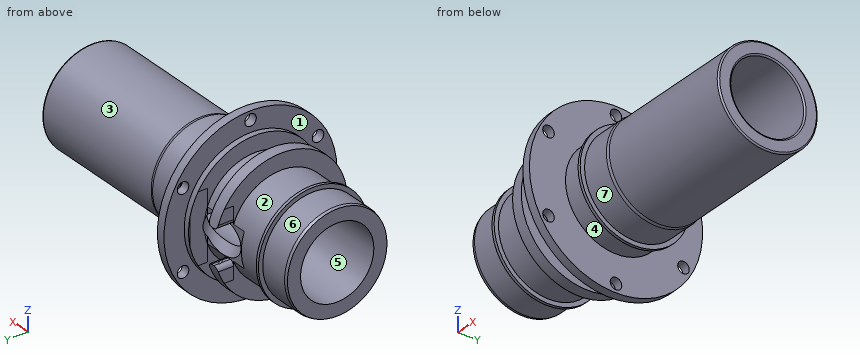
from build123d import *
from build123d.topology import SkipClean

# Parameters (mm, degrees)
SKETCH2_R          = 2
CUT_EXTRUDE1_DEPTH = 92.660037639
CUT_EXTRUDE2_DEPTH = 6.025391911


# Read off the part's stored shape, not the designer's step: Cut-Extrude2
with BuildPart() as part:
    # Sketch1 → Revolve1 (revolve)
    with BuildSketch(Plane.XY, mode=Mode.PRIVATE) as revolve1_sk:
        with BuildLine():
            Line((-1.5, 17.5), (6.5, 17.5))
            Line((6.5, 17.5), (6.5, 23))
            Line((6.5, 23), (8.5, 23))
            Line((8.5, 23), (8.5, 30))
            Line((8.5, 30), (11.5, 30))
            Line((11.5, 30), (11.5, 17.5))
            Line((11.5, 17.5), (19.25, 17.5))
            Line((19.25, 17.5), (19.25, 19))
            Line((19.25, 19), (20.25, 19))
            Line((20.25, 19), (20.25, 17.5))
            Line((20.25, 17.5), (30.25, 17.5))
            Line((30.25, 17.5), (31.25, 17.25))
            Line((31.25, 17.25), (80.75, 17.25))
            ThreePointArc((80.75, 17.25), (81.103553391, 17.103553391), (81.25, 16.75))
            Line((81.25, 16.75), (81.25, 13.2))
            ThreePointArc((81.25, 13.2), (81.103553391, 12.846446609), (80.75, 12.7))
            Line((80.75, 12.7), (-31.25, 12.7))
            Line((-31.25, 12.7), (-31.25, 17.25))
            Line((-31.25, 17.25), (-30.25, 17.5))
            Line((-30.25, 17.5), (-20.25, 17.5))
            Line((-20.25, 17.5), (-20.25, 19))
            Line((-20.25, 19), (-19.25, 19))
            Line((-19.25, 19), (-19.25, 17.5))
            Line((-19.25, 17.5), (-5.5, 17.5))
            Line((-5.5, 17.5), (-5.5, 23))
            Line((-5.5, 23), (-1.5, 23))
            Line((-1.5, 23), (-1.5, 17.5))
        make_face()
    revolve(revolve1_sk.sketch.rotate(Axis((-31.25, 0, 0), (1, 0, 0)), 180), axis=Axis((-31.25, 0, 0), (1, 0, 0)))

    # Sketch2 → Cut-Extrude1 (cut, through all)
    with BuildSketch(Plane(origin=(0, 0, 0), x_dir=(0, 0, -1), z_dir=(1, 0, 0))):
        with Locations(Location((27, 0, 0), (0, 0, 270))):
            Circle(SKETCH2_R)
        with Locations(Location((13.5, -23.382685902, 0), (0, 0, 270))):
            Circle(SKETCH2_R)
        with Locations(Location((-13.5, -23.382685902, 0), (0, 0, 270))):
            Circle(SKETCH2_R)
        with Locations(Location((-27, 0, 0), (0, 0, 270))):
            Circle(SKETCH2_R)
        with Locations(Location((-13.5, 23.382685902, 0), (0, 0, 270))):
            Circle(SKETCH2_R)
        with Locations(Location((13.5, 23.382685902, 0), (0, 0, 270))):
            Circle(SKETCH2_R)
    extrude(amount=CUT_EXTRUDE1_DEPTH, mode=Mode.SUBTRACT)

    # Sketch3 → Cut-Revolve1 (revolve, cut)
    with BuildSketch(Plane.XY):
        Polygon((16, 0), (-16.947446606, 32.947446606), (-21.190087293, 28.704805919), (11.757359313, -4.242640687), align=None)
    revolve(axis=Axis((-23.931199794, 39.931199794, 0), (0.7071067811865516, -0.7071067811865436, 0)), mode=Mode.SUBTRACT)

    # Cut-Extrude2 outline → Cut-Extrude2 (cut)
    with SkipClean():  # the faces are left unmerged after this step: merging them gives an invalid solid
        with BuildSketch(Plane(origin=(0, 16.455853693, 0), x_dir=(1, 0, 0), z_dir=(0, 1, 0))):
            with BuildLine():
                Line((-2.992126028, 5.992167254), (-3.992126028, 5.986917867))
                ThreePointArc((-3.992126028, 5.986917867), (-5.057872639, 6.423456803), (-5.5, 7.4868972))
                Line((-5.5, 7.4868972), (-5.5, 11.85382039))
                Line((-5.5, 11.85382039), (-10.416830721, 11.85382039))
                Line((-10.416830721, 11.85382039), (-10.416830721, 5.95439999))
                Line((-10.416830721, 5.95439999), (-10.416830721, -5.95439999))
                Line((-10.416830721, -5.95439999), (-10.416830721, -11.85382039))
                Line((-10.416830721, -11.85382039), (-5.5, -11.85382039))
                Line((-5.5, -11.85382039), (-5.5, -7.4868972))
                ThreePointArc((-5.5, -7.4868972), (-5.057872639, -6.423456803), (-3.992126028, -5.986917867))
                Line((-3.992126028, -5.986917867), (-2.992126028, -5.992167254))
                ThreePointArc((-2.992126028, -5.992167254), (-1.936559603, -6.434273947), (-1.5, -7.492146587))
                Line((-1.5, -7.492146587), (-1.5, -11.85382039))
                Line((-1.5, -11.85382039), (6.5, -11.85382039))
                Line((6.5, -11.85382039), (6.5, 11.85382039))
                Line((6.5, 11.85382039), (-1.5, 11.85382039))
                Line((-1.5, 11.85382039), (-1.5, 7.492146587))
                ThreePointArc((-1.5, 7.492146587), (-1.936559603, 6.434273947), (-2.992126028, 5.992167254))
            make_face()
        extrude(amount=CUT_EXTRUDE2_DEPTH, mode=Mode.SUBTRACT)


solid = part.part
Part model, mm, in its own coordinate system. Face numbers are marked on the shaded views. A direction names the side the tool comes from. Coordinates: 2 decimals unless noted, no trailing zeros. Order: outer loops, then holes, each group sorted by start corner. A loop starts at its lowest first (then second) coordinate and runs counter-clockwise, first axis right, second up. Notation, with made-up numbers: M 12,-29.75 L 42,-29.75 A13 cw 42,-22.75 Z; hole C 50.5,-12 d3. An arc over 180 degrees is marked long. Use a Markdown table: item, result.
(1) Cut at B-B on x = 41.5. Write the cut outline in (y, z).
A:
| item | result |
|---|---|
| outline | C 0,0 d34.5; hole C 0,0 d25.4 |
(2) Probe L1, parallel to Z at x = 10.35, y = 0; L2, parallel to X at y = 19.5, z = 8.5; L3, parallel to Z at x = 35.5, y = 0. List the from-to ranges inside material, lowest first.
A:
| item | result |
|---|---|
| L1 | z = -30 to -29, -25 to -12.7, 12.7 to 25, 29 to 30 |
| L2 | x = -5.5 to -1.5, 6.5 to 11.5 |
| L3 | z = -17.25 to -12.7, 12.7 to 17.25 |
(3) Cut at A-A on z = -27. Write the cut outline in (x, y), then the cut area to 3 significant figures.
A:
| item | result |
|---|---|
| outline | M 8.5,-13.08 L 11.5,-13.08 L 11.5,-2 L 8.5,-2 Z; M 8.5,2 L 11.5,2 L 11.5,13.08 L 8.5,13.08 Z |
| area | 66.5 mm^2 |
(4) Cut at D-D on x = -24. Write the cut outline in (y, z), then the cut area to 3 significant figures.
A:
| item | result |
|---|---|
| outline | C 0,0 d35; hole C 0,0 d25.4 |
| area | 455 mm^2 |
(5) Pull direction X, two halves, no side cores. Call the marked faces 1, 2 and 3: released by +X, released by -X, zero draft, split by the parting line, or undercut.
A:
| item | result |
|---|---|
| face 1 | released by -X |
| face 2 | undercut |
| face 3 | zero draft |
(6) Cut at C-C on z = -21. Write the cut outline in (x, y).
A:
| item | result |
|---|---|
| outline | M -5.5,-9.38 L -1.5,-9.38 L -1.5,9.38 L -5.5,9.38 Z; M 6.5,-9.38 L 8.5,-9.38 L 8.5,-21.42 L 11.5,-21.42 L 11.5,21.42 L 8.5,21.42 L 8.5,9.38 L 6.5,9.38 Z |
(7) Tool access for the marked faces 4, 5, 6 and 7: list every direction of +Z, -Z, +X, -X, +Y, -Y with a clear straight run to the whole face (end or side of a thin tool).
A:
| item | result |
|---|---|
| face 4 | none |
| face 5 | +X, -X |
| face 6 | -X |
| face 7 | +X |
(8) Flat gauge pins, fed straight in: pin 1 (2.5 mm diameter, centred on y = 23.38, z = -13.5, fed in from +X); pin 2 (6.5 mm diameter, centred on y = 0, z = -27, fed in from -X); pin 3 (12 mm diameter, centred on y = 21.5, z = -11, fed in from +X); pin 4 (1 mm diameter, centred on y = 17, z = -3.5, fed in from -X). Where does each tip first touch, or does it go through?
A:
| item | result |
|---|---|
| pin 1 | passes through |
| pin 2 | stops at x = 8.5 |
| pin 3 | stops at x = 20.25 |
| pin 4 | stops at x = -31.25 |
